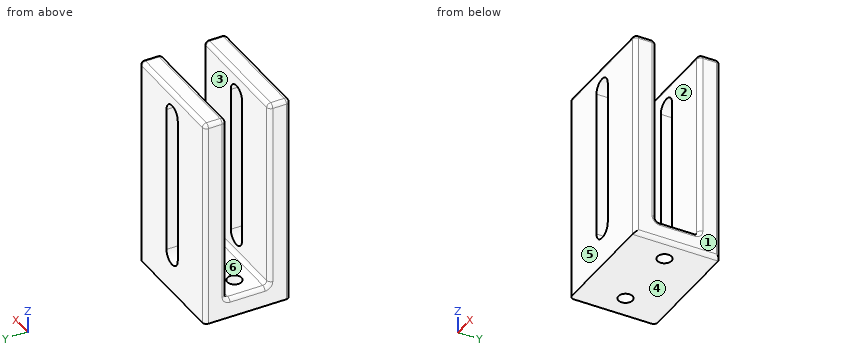
```python
from build123d import *

# Parameters (mm, degrees)
F0_W     = 30
F0_H     = 54
F1_DEPTH = 11
F2_W     = 30
F2_H     = 11
F3_DEPTH = 49
F4_R     = 1.825
F5_DEPTH = 5
F6_F1_R  = 1
F6_F2_R  = 1


with BuildPart() as f1:
    # F0 (on Front) → F1 (new body, symmetric)
    with BuildSketch(Plane.XZ):
        with Locations((-15, 27)):
            Rectangle(F0_W, F0_H)
        with BuildLine():
            Line((-17.6, 10), (-17.6, 48))
            ThreePointArc((-17.6, 48), (-15, 50.6), (-12.4, 48))
            Line((-12.4, 48), (-12.4, 10))
            ThreePointArc((-12.4, 10), (-15, 7.4), (-17.6, 10))
        make_face(mode=Mode.SUBTRACT)
    extrude(amount=F1_DEPTH, both=True)

    # F2 (on face) → F3 (cut, through all)
    with BuildSketch(Plane.XY.offset(54)):
        with Locations((-15, 0)):
            Rectangle(F2_W, F2_H)
    extrude(amount=-F3_DEPTH, mode=Mode.SUBTRACT)

    # F4 (on Top) → F5 (cut, through all)
    with BuildSketch(Plane.XY):
        with Locations((-24, 0)):
            Circle(F4_R)
        with Locations((-6, 0)):
            Circle(F4_R)
    extrude(amount=F5_DEPTH, mode=Mode.SUBTRACT)

    # F6: fillet of radius 1 on 19 edges, made by hand

    # F6_f1
    f6_f1_edges = [f1.edges().sort_by_distance(p)[0] for p in [
        (-15, -5.5, 5),
        (-15, 5.5, 5),
    ]]
    fillet(f6_f1_edges, radius=F6_F1_R)

    # F6_f2
    f6_f2_edges = [f1.edges().sort_by_distance(p)[0] for p in [
        (-30, -11, 27),
        (-30, -5.5, 30),
        (-30, 5.5, 30),
        (0, 5.5, 30),
        (0, 11, 27),
        (-30, 11, 27),
        (-15, 11, 54),
        (-15, 5.5, 54),
        (-15, -11, 54),
        (-15, -5.5, 54),
        (0, -5.5, 30),
        (0, -11, 27),
        (0, -8.25, 54),
        (0, 8.25, 54),
        (0, 0, 0),
        (-30, -8.25, 54),
        (-30, 8.25, 54),
        (0, -5.2071067812, 5.2928932188),
        (0, 5.2071067812, 5.2928932188),
        (-30, 5.2071067812, 5.2928932188),
        (-30, -5.2071067812, 5.2928932188),
    ]]
    fillet(f6_f2_edges, radius=F6_F2_R)


solid = f1.part
```
Check sheet for the modelled part. Datum: model origin and axes. Units: mm. Face numbers are marked on the shaded views. A direction names the side the tool comes from. Round coordinates to 2 decimals unless told otherwise and drop trailing zeros. Loops run counter-clockwise (first coordinate to the right, second up) from the corner with the lowest first, then second, coordinate; pieces in that order, holes last. Notation, with made-up numbers: (-29, -35) -> (-14, -35) arc R14 ccw to (-14, -15) -> close; hole circle Ø9 at (15, 42). An arc over 180 degrees is marked (long way). Answer in a Markdown table with one row per item.
Q1. Go/stop test with a flat-tipped pin: P1, Ø2, axis at x = -12, y = 0, coming from the +Z side. Record where the tip stops, or that it passes through.
Data:
| item | result |
|---|---|
| P1 | stops at z = 5 |
Q2. Sectioned sample at D-D on y = 0. Enter the section's corners in (x, z) (3 decimals).
Data:
| item | result |
|---|---|
| outline | (-30, 0) -> (-25.825, 0) -> (-25.825, 5) -> (-29, 5) arc R1 ccw to (-30, 4) -> close; (-22.175, 0) -> (-7.825, 0) -> (-7.825, 5) -> (-22.175, 5) -> close; (-4.175, 0) -> (-1, 0) arc R1 ccw to (0, 1) -> (0, 4) arc R1 ccw to (-1, 5) -> (-4.175, 5) -> close |
Q3. Thickness scan on L1, parallel to Y at x = -22.25, z = 48; L2, parallel to Y at x = -24, z = 3.85 (3 decimals); L3, parallel to X at y = 6.5, z = 29. Record the ranges inside material, lowest first.
Data:
| item | result |
|---|---|
| L1 | y = -11 to -5.5, 5.5 to 11 |
| L2 | y = -11 to -1.825, 1.825 to 11 |
| L3 | x = -30 to -17.6, -12.4 to 0 |
Q4. Release check for a two-part mould opening along Y. For the marked faces 3, 4, 5 and 6 record: released by +Y, released by -Y, zero draft, split by the parting line, or undercut.
Data:
| item | result |
|---|---|
| face 3 | undercut |
| face 4 | zero draft |
| face 5 | released by -Y |
| face 6 | undercut |
Q5. Set-up check for the marked faces 1 and 2: record each of +Z, -Z, +X, -X, +Y, -Y from which the full face is reachable in a straight line by a thin tool's end or side.
Data:
| item | result |
|---|---|
| face 1 | +Z, -Z, +X, +Y, -Y |
| face 2 | +Z, +X, -X |
Q6. Sectioned sample at C-C on z = 39. Enter the section's corners in (x, y), then the cut area to 3 significant figures.
Data:
| item | result |
|---|---|
| outline | (-30, -10) arc R1 ccw to (-29, -11) -> (-17.6, -11) -> (-17.6, -5.5) -> (-29, -5.5) arc R1 ccw to (-30, -6.5) -> close; (-30, 6.5) arc R1 ccw to (-29, 5.5) -> (-17.6, 5.5) -> (-17.6, 11) -> (-29, 11) arc R1 ccw to (-30, 10) -> close; (-12.4, -11) -> (-1, -11) arc R1 ccw to (0, -10) -> (0, -6.5) arc R1 ccw to (-1, -5.5) -> (-12.4, -5.5) -> close; (-12.4, 5.5) -> (-1, 5.5) arc R1 ccw to (0, 6.5) -> (0, 10) arc R1 ccw to (-1, 11) -> (-12.4, 11) -> close |
| area | 271 mm^2 |
Q7. Sectioned sample at B-B on x = -6. Enter the section's corners in (y, z) (3 decimals).
Data:
| item | result |
|---|---|
| outline | (-11, 0) -> (-1.825, 0) -> (-1.825, 5) -> (-4.5, 5) arc R1 cw to (-5.5, 6) -> (-5.5, 53) arc R1 ccw to (-6.5, 54) -> (-10, 54) arc R1 ccw to (-11, 53) -> close; (1.825, 0) -> (11, 0) -> (11, 53) arc R1 ccw to (10, 54) -> (6.5, 54) arc R1 ccw to (5.5, 53) -> (5.5, 6) arc R1 cw to (4.5, 5) -> (1.825, 5) -> close |
Q8. Sectioned sample at A-A on x = -15. Enter the section's corners in (y, z), then the cut area to 3 significant figures.
Data:
| item | result |
|---|---|
| outline | (-11, 0) -> (11, 0) -> (11, 7.4) -> (5.5, 7.4) -> (5.5, 6) arc R1 cw to (4.5, 5) -> (-4.5, 5) arc R1 cw to (-5.5, 6) -> (-5.5, 7.4) -> (-11, 7.4) -> close; (-11, 50.6) -> (-5.5, 50.6) -> (-5.5, 53) arc R1 ccw to (-6.5, 54) -> (-10, 54) arc R1 ccw to (-11, 53) -> close; (5.5, 50.6) -> (11, 50.6) -> (11, 53) arc R1 ccw to (10, 54) -> (6.5, 54) arc R1 ccw to (5.5, 53) -> close |
| area | 173 mm^2 |
